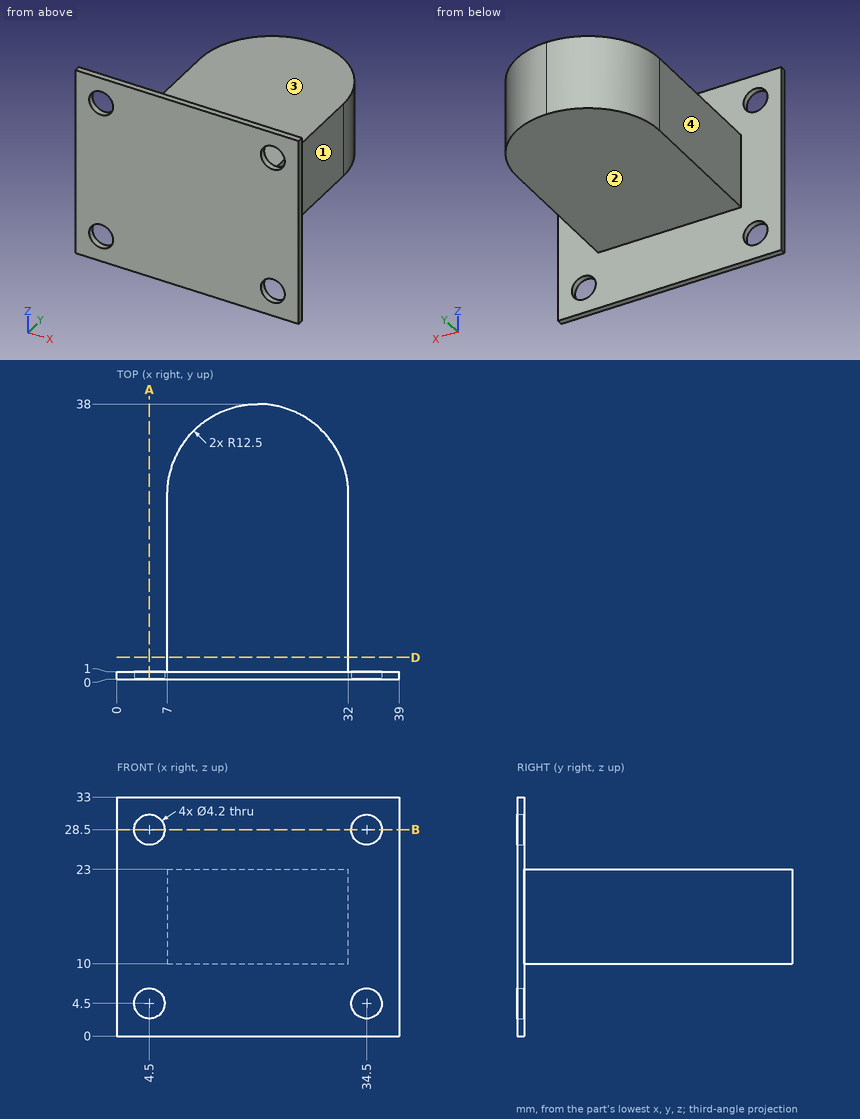
Answer from the drawing. Dimensions are ordinates in mm from the lowest x, y and z of the part. A direction names the side the tool comes from. Give positions to 0.01 mm unless a question says otherwise; leave off trailing zeros. Order: outer loops, then holes, each group sorted by start corner. A loop starts at its lowest first (then second) coordinate and runs counter-clockwise, first axis right, second up.
(1) Find section A-A (x = 4.5). Give the vertices of the cut face in (y, z), plus the area to 3 significant figures.
(2) Find section B-B (z = 28.5). Give the vertices of the cut face in (x, y), plus the area to 3 significant figures.
(3) Straight lines are drawn through the part: L1, parallel to X at y = 0.5, z = 28.5; L2, parallel to Z at x = 19, y = 22; L3, parallel to X at y = 20, z = 13.5. For each, find the intervals that lie inside material, in ascending order.
(4) For the marked faces 1, 2, 3 and 4, determine the directions among +Z, -Z, +X, -X, +Y, -Y from which every point of the face is accessible in a straight line to the end or side of a thin tool.
(5) Find section D-D (y = 3). Give the vertices of the cut face in (x, z), plus the area to 3 significant figures.
(6) Given pin 1 (1 mm diameter, centred on x = 24.5, y = 14.5, fed in from +Z); pin 2 (1.5 mm diameter, centred on x = 21, y = 34, fed in from -Z); pin 3 (6.5 mm diameter, centred on y = 17, z = 17, fed in from +X), each flat-ended and moving along its own axis, determine where each tip first touches the part or whether it passes through.
Result sheet:
1. outline: (0, 0) - (1, 0) - (1, 2.4) - (0, 2.4) - close; (0, 6.6) - (1, 6.6) - (1, 26.4) - (0, 26.4) - close; (0, 30.6) - (1, 30.6) - (1, 33) - (0, 33) - close
1. area: 24.6 mm2
2. outline: (0, 0) - (2.4, 0) - (2.4, 1) - (0, 1) - close; (6.6, 0) - (32.4, 0) - (32.4, 1) - (6.6, 1) - close; (36.6, 0) - (39, 0) - (39, 1) - (36.6, 1) - close
2. area: 30.6 mm2
3. L1: x = 0 to 2.4, 6.6 to 32.4, 36.6 to 39
3. L2: z = 10 to 23
3. L3: x = 7 to 32
4. face 1: +Z, -Z, +X, +Y
4. face 2: -Z, +X, -X, +Y
4. face 3: +Z, +X, -X, +Y
4. face 4: +Z, -Z, -X, +Y
5. outline: (7, 10) - (32, 10) - (32, 23) - (7, 23) - close
5. area: 325 mm2
6. pin 1: stops at z = 23
6. pin 2: stops at z = 10
6. pin 3: stops at x = 32
